```python
from build123d import *

# Parameters (mm, degrees)
F0_R     = 1.4986
F1_DEPTH = 6.35
F2_SIZE  = 0.9906
F0_R_2   = 1.524
F3_DEPTH = 3.81
F5_DEPTH = 5.08
F7_DEPTH = 5.08
F8_R     = 3.81


with BuildPart() as f1:
    # F0 (on Front) → F1 (new body)
    with BuildSketch(Plane.XZ):
        with BuildLine():
            Line((-36.0867052997, 143.2092670372), (-42.4367052997, 143.2092670372))
            Line((-42.4367052997, 143.2092670372), (-42.4367052997, 52.8312826116))
            ThreePointArc((-42.4367052997, 52.8312826116), (-43.703811406, 49.7245670372), (-42.4367052997, 46.6178514628))
            Line((-42.4367052997, 46.6178514628), (-42.4367052997, 3.2298670372))
            Line((-42.4367052997, 3.2298670372), (-36.0867052997, 3.2298670372))
            Line((-36.0867052997, 3.2298670372), (-36.0867052997, 38.2945670372))
            ThreePointArc((-36.0867052997, 38.2945670372), (-34.5988077481, 41.8866694856), (-31.0067052997, 43.3745670372))
            Line((-31.0067052997, 43.3745670372), (-13.2267052997, 43.3745670372))
            ThreePointArc((-13.2267052997, 43.3745670372), (-9.6346028513, 41.8866694856), (-8.1467052997, 38.2945670372))
            Line((-8.1467052997, 38.2945670372), (-8.1467052997, 3.2298670372))
            Line((-8.1467052997, 3.2298670372), (-1.7967052997, 3.2298670372))
            Line((-1.7967052997, 3.2298670372), (-1.7967052997, 46.6178514628))
            ThreePointArc((-1.7967052997, 46.6178514628), (-0.5295991933, 49.7245670372), (-1.7967052997, 52.8312826116))
            Line((-1.7967052997, 52.8312826116), (-1.7967052997, 143.2092670372))
            Line((-1.7967052997, 143.2092670372), (-8.1467052997, 143.2092670372))
            Line((-8.1467052997, 143.2092670372), (-8.1467052997, 61.1545671391))
            ThreePointArc((-8.1467052997, 61.1545671391), (-9.6346028513, 57.5624646907), (-13.2267052997, 56.0745671391))
            Line((-13.2267052997, 56.0745671391), (-31.0067052997, 56.0745671391))
            ThreePointArc((-31.0067052997, 56.0745671391), (-34.5988077481, 57.5624646907), (-36.0867052997, 61.1545671391))
            Line((-36.0867052997, 61.1545671391), (-36.0867052997, 143.2092670372))
        make_face()
        with Locations((-39.2617052997, 7.3065670372)):
            Circle(F0_R, mode=Mode.SUBTRACT)
        with BuildLine():
            ThreePointArc((-40.7603052997, 48.2259670372), (-42.2589052997, 49.7245670372), (-40.7603052997, 51.2231670372))
            Line((-40.7603052997, 51.2231670372), (-37.7631052997, 51.2231670372))
            ThreePointArc((-37.7631052997, 51.2231670372), (-36.2645052997, 49.7245670372), (-37.7631052997, 48.2259670372))
            Line((-37.7631052997, 48.2259670372), (-40.7603052997, 48.2259670372))
        make_face(mode=Mode.SUBTRACT)
        with Locations((-4.9717052997, 7.3065670372)):
            Circle(F0_R, mode=Mode.SUBTRACT)
        with BuildLine():
            ThreePointArc((-6.4703052997, 48.2259670372), (-7.9689052997, 49.7245670372), (-6.4703052997, 51.2231670372))
            Line((-6.4703052997, 51.2231670372), (-3.4731052997, 51.2231670372))
            ThreePointArc((-3.4731052997, 51.2231670372), (-1.9745052997, 49.7245670372), (-3.4731052997, 48.2259670372))
            Line((-3.4731052997, 48.2259670372), (-6.4703052997, 48.2259670372))
        make_face(mode=Mode.SUBTRACT)
        with Locations((-39.2617052997, 139.1325670372)):
            Circle(F0_R, mode=Mode.SUBTRACT)
        with Locations((-4.9717052997, 139.1325670372)):
            Circle(F0_R, mode=Mode.SUBTRACT)
    extrude(amount=F1_DEPTH)

    # F2
    f2_edges = [f1.edges().sort_by_distance(p)[0] for p in [
        (-40.760305, -6.35, 7.306567),
        (-36.264505, -6.35, 49.724567),
        (-40.760305, -6.35, 139.132567),
        (-4.971705, -6.35, 48.225967),
        (-6.470305, -6.35, 7.306567),
        (-6.470305, -6.35, 139.132567),
    ]]
    chamfer(f2_edges, length=F2_SIZE)

    # F0 (on Front) → F3 (join)
    with BuildSketch(Plane.XZ):
        with BuildLine():
            Line((-22.1167052997, 68.3935671391), (-36.0867052997, 61.1545671391))
            ThreePointArc((-36.0867052997, 61.1545671391), (-34.5988077481, 57.5624646907), (-31.0067052997, 56.0745671391))
            Line((-31.0067052997, 56.0745671391), (-22.1167052997, 58.9955671391))
            Line((-22.1167052997, 58.9955671391), (-13.2267052997, 56.0745671391))
            ThreePointArc((-13.2267052997, 56.0745671391), (-9.6346028513, 57.5624646907), (-8.1467052997, 61.1545671391))
            Line((-8.1467052997, 61.1545671391), (-22.1167052997, 68.3935671391))
        make_face()
        with Locations((-22.1167052997, 63.6945671391)):
            Circle(F0_R_2, mode=Mode.SUBTRACT)
    extrude(amount=F3_DEPTH)

    # F4 (on face) → F5 (cut)
    with BuildSketch(Plane(origin=(-8.1467052997, 0, 0), x_dir=(0, -1, 0), z_dir=(-1, 0, 0))):
        with BuildLine():
            ThreePointArc((4.445, 97.2352670372), (3.1430896424, 100.3783566796), (0, 101.6802670372))
            Line((0, 101.6802670372), (0, 97.2352670372))
            Line((0, 97.2352670372), (0, 92.7902670372))
            ThreePointArc((0, 92.7902670372), (3.1430896424, 94.0921773948), (4.445, 97.2352670372))
        make_face()
        with BuildLine():
            ThreePointArc((4.445, 66.2472670372), (3.1430896424, 69.3903566796), (0, 70.6922670372))
            Line((0, 70.6922670372), (0, 66.2472670372))
            Line((0, 66.2472670372), (0, 61.8022670372))
            ThreePointArc((0, 61.8022670372), (3.1430896424, 63.1041773948), (4.445, 66.2472670372))
        make_face()
    extrude(amount=-F5_DEPTH, mode=Mode.SUBTRACT)

    # F6 (on face) → F7 (cut)
    with BuildSketch(Plane.YZ.offset(-36.0867052997)):
        with BuildLine():
            Line((0, 97.2352670372), (0, 101.6802670372))
            ThreePointArc((0, 101.6802670372), (-4.445, 97.2352670372), (0, 92.7902670372))
            Line((0, 92.7902670372), (0, 97.2352670372))
        make_face()
        with BuildLine():
            Line((0, 66.2472670372), (0, 70.6922670372))
            ThreePointArc((0, 70.6922670372), (-4.445, 66.2472670372), (0, 61.8022670372))
            Line((0, 61.8022670372), (0, 66.2472670372))
        make_face()
    extrude(amount=-F7_DEPTH, mode=Mode.SUBTRACT)

    # F8
    f8_edges = [f1.edges().sort_by_distance(p)[0] for p in [
        (-22.116705, -1.905, 68.393567),
    ]]
    fillet(f8_edges, radius=F8_R)


solid = f1.part
```
The listing builds one solid part. Answer for the finished solid, in the listing's coordinates (mm). A direction names the side the tool comes from. Give positions to 0.01 mm unless a question says otherwise; leave off trailing zeros. Loops run counter-clockwise (first coordinate to the right, second up) from the corner with the lowest first, then second, coordinate; pieces in that order, holes last. Notation, with made-up numbers: (50, 44) - (84, 44) arc R20 cw to (84, 76) - close; hole circle Ø9 at (65.25, 86). An arc over 180 degrees is marked (long way). Return JSON: item names as keys, results as strings. Group by question number.
1. Straight lines are drawn through the part: line 1 (X direction, y = -5.25, z = 96.5); line 2 (Z direction, x = -41, y = -2); line 3 (Z direction, x = -5, y = -1.25). For each, find the intervals that lie inside material, in ascending order. Write a range as [from, to].
2. Find section C-C (y = -1.25). State how many separate pieces and enclosed holes the cut face has, then the cut area to 3 significant figures.
3. Given pin 1 Ø3 at (y, z) = (-2.5, 100.5) entering from -X; pin 2 Ø3.5 at (x, z) = (-4.97, 7.31) entering from -Y; pin 3 Ø5 at (x, z) = (-20.5, 71.5) entering from -Y; pin 4 Ø1.9 at (y, z) = (-4.5, 20.5) entering from +X, each flat-ended and moving along its own axis, determine where each tip first touches the part or whether it passes through.
4. Which of the six approach directions +Z, -Z, +X, -X, +Y, -Y give full straight-line access (tool end or side, diameter ignored) to faces 1 (the flat face through (-39, -3, 48.226)), 2 (the flat face through (-42.437, -3, 99)), 3 (the cylindrical face through (-38.591, -4.444, 97.333)), 4 (the conical face through (-36.093, -5.531, 49.761))?
5. Find section A-A (z = 82). Write down the section's boundary in (x, y).
6. Find section B-B (x = -12). Write down the section's boundary in (y, z).
7. Determine the mould class of faces 5 (the cylindrical face through (-34.638, -3.131, 41.847)), 6 (the flat face through (-36.087, -3, 21)), 7 (the conical face through (-42.4, -5.5, 49.7)) for opening direction Z: pulls with the +Z half, pulls with the -Z half, needs draft (parallel to the pull), parting line crosses it, or undercut.
Verdict:
{
 "1": {"line 1": "x = [-42.44, -36.09], [-8.15, -1.8]", "line 2": "z = [3.23, 48.25], [51.2, 62.28], [70.22, 93.27], [101.2, 143.21]", "line 3": "z = [3.23, 5.81], [8.8, 48.23], [51.22, 61.98], [70.51, 92.97], [101.5, 137.63], [140.63, 143.21]"},
 "2": {"separate pieces": "1", "enclosed holes": "8", "area": "2,130 mm^2"},
 "3": {"pin 1": "stops at x = -42.44", "pin 2": "stops at y = -5.61", "pin 3": "passes through", "pin 4": "stops at x = -1.8"},
 "4": {"face 1": "+Y, -Y", "face 2": "+Z, -X, +Y, -Y", "face 3": "+Y", "face 4": "-Y"},
 "5": {"outline": "(-42.44, -6.35) - (-36.09, -6.35) - (-36.09, 0) - (-42.44, 0) - close; (-8.15, -6.35) - (-1.8, -6.35) - (-1.8, 0) - (-8.15, 0) - close"},
 "6": {"outline": "(-6.35, 43.22) - (0, 43.22) - (0, 63.15) - (-3.81, 63.15) - (-3.81, 56.22) - (-6.35, 56.22) - close"},
 "7": {"face 5": "pulls with the -Z half", "face 6": "needs draft", "face 7": "undercut"}
}
